from build123d import *

# Parameters (mm, degrees)
EXTRUDE_1_DEPTH          = 3
SKETCH_2_R               = 7.1
SKETCH_2_R_2             = 5.05
CUT_EXTRUDE_1_DEPTH      = 10
SKETCH_3_R               = 2.55
CUT_EXTRUDE_2_DEPTH      = 10
PATTERN_CIRCULAR_1_COUNT = 3
CHAMFER_1_SIZE           = 0.5
SKETCH_4_R               = 8.1
CUT_EXTRUDE_3_DEPTH      = 1


with BuildPart() as part:
    # 草图1 → 凸台-拉伸1 (new body)
    with BuildSketch(Plane(origin=(0, 0, 0), x_dir=(0, 0, -1), z_dir=(1, 0, 0))):
        with BuildLine():
            ThreePointArc((6.766526321, -35.674580026), (11.667792815, -16.687604516), (9.596471541, 2.812069339))
            ThreePointArc((9.596471541, 2.812069339), (0.889352151, 9.960374127), (-8.946463525, 4.467750037))
            Line((-8.946463525, 4.467750037), (-22.078912993, -21.829374729))
            ThreePointArc((-22.078912993, -21.829374729), (-14.688022315, -43.402261843), (6.766526321, -35.674580026))
        make_face()
    extrude(amount=EXTRUDE_1_DEPTH)

    # 草图2 → 切除-拉伸1 (cut)
    with BuildSketch(Plane.ZY):
        Circle(SKETCH_2_R)
        with Locations((7.764571353, -28.977774789)):
            Circle(SKETCH_2_R_2)
    extrude(amount=-CUT_EXTRUDE_1_DEPTH, mode=Mode.SUBTRACT)

    # 草图3 → 切除-拉伸2 (cut)
    with BuildSketch(Plane.ZY):
        with Locations((5.176380902, -19.318516526)):
            Circle(SKETCH_3_R)
    cut_extrude_2 = extrude(amount=-CUT_EXTRUDE_2_DEPTH, mode=Mode.SUBTRACT)

    # 阵列(圆周)1: 切除-拉伸2 ×3 about axis
    pattern_circular_1_axis = Axis((0, -28.977774789, 7.764571353), (1, 0, 0))
    for i in range(1, PATTERN_CIRCULAR_1_COUNT):
        add(cut_extrude_2.rotate(pattern_circular_1_axis, i * 360 / PATTERN_CIRCULAR_1_COUNT), mode=Mode.SUBTRACT)

    # 倒角1
    chamfer_1_edges = [part.edges().sort_by_distance(p)[0] for p in [
        (3, -28.977774789, 2.714571353),
    ]]
    chamfer(chamfer_1_edges, length=CHAMFER_1_SIZE)

    # 草图4 → 切除-拉伸3 (cut)
    with BuildSketch(Plane.ZY.offset(-3)):
        Circle(SKETCH_4_R)
    extrude(amount=CUT_EXTRUDE_3_DEPTH, mode=Mode.SUBTRACT)


solid = part.part
Read the model definition and answer for the solid it produces. Units are mm, in the model's axes. A direction names the side the tool comes from. Give positions to 0.01 mm unless a question says otherwise; leave off trailing zeros. Write each loop counter-clockwise with the first axis right and the second up, starting at its lowest first coordinate (ties: lowest second). Pieces come first, ordered by that corner, then holes. Notation, with made-up numbers: (-8, 29.25) - (34, 29.25) arc R10 cw to (34, 35.25) - close; hole circle Ø10 at (72, 26). An arc over 180 degrees is marked (long way). Use CSV: the item, a comma, the result in double quotes. Start each with the question number.
(1) Given P1, Ø4, axis at y = -21, z = 14, coming from the -X side; P2, Ø1.5, axis at x = 2, z = -5.5, coming from the +Y side; P3, Ø1, axis at x = 1.5, z = -4, coming from the -Y side, each flat-ended and moving along its own axis, determine where each tip first touches the part or whether it passes through.
(2) Find section D-D (z = -6). Give the vertices of the cut face in (x, y), plus the area to 3 significant figures.
(3) Determine the mould class of faces 3 (the cylindrical face through (1.479, 9.944, -1.056)), 4 (the flat face through (1.479, -8.497, 15.421)), 5 (the cylindrical face through (1.479, -16.963, -11.647)), 6 (the cylindrical face through (1.479, -29.416, 18.795)) for opening direction Z: +Z half, -Z half, draft (parallel to the pull), parting line (faces both ways), or undercut.
(4) Find section C-C (x = 0.55). Give the vertices of the cut face in (y, z).
(5) Consider line 1 along Y through (x, z) = (2.15, 3.5); line 2 along Y through (x, z) = (1.05, 4.5); line 3 along Y through (x, z) = (1.95, -1). Determine where each line is inside the solid, lowest interval first.
(6) Find section A-A (y = 0). Give the vertices of the cut face in (x, z).
(7) Find section B-B (z = 0). Give the vertices of the cut face in (x, y), plus the area to 3 significant figures.
(8) For faces 1 (the cylindrical face through (0.99, 7.04, -0.92)), 2 (the cylindrical face through (2.507, -7.907, -1.756)), determine the directions among +Z, -Z, +X, -X, +Y, -Y from which every point of the face is accessible in a straight line to the end or side of a thin tool.
Findings below:
1,P1,"x = 0"
1,P2,"y = 8.8"
1,P3,"y = -40.34"
2,outline,"(0, -37.13) - (3, -37.13) - (3, -5.44) - (2, -5.44) - (2, -3.8) - (0, -3.8) - close; (0, 3.8) - (2, 3.8) - (2, 5.44) - (3, 5.44) - (3, 8) - (0, 8) - close"
2,area,"109 mm2"
3,face 3,"parting line"
3,face 4,"+Z half"
3,face 5,"-Z half"
3,face 6,"undercut"
4,outline,"(-35.67, -6.77) arc R55 ccw to (2.81, -9.6) arc R10 ccw to (4.47, 8.95) - (-21.83, 22.08) arc R16 ccw (long way) to start; hole circle Ø5.1 at (-36.05, 0.69); hole circle Ø5.1 at (-31.57, 17.42); hole circle Ø10.1 at (-28.98, 7.76); hole circle Ø5.1 at (-19.32, 5.18); hole circle Ø14.2 at (0, 0)"
5,line 1,"-44.4 to -31.68, -26.27 to -21.24, -17.4 to -7.3, 7.3 to 9.37"
5,line 2,"-44.64 to -32.83, -25.12 to -21.78, -16.86 to -5.49, 5.49 to 8.93"
5,line 3,"-42.36 to -37.96, -34.14 to -7.03, 7.03 to 9.95"
6,outline,"(0, -10.34) - (3, -10.34) - (3, -8.1) - (2, -8.1) - (2, -7.1) - (0, -7.1) - close; (0, 7.1) - (2, 7.1) - (2, 8.1) - (3, 8.1) - (3, 11.18) - (0, 11.18) - close"
7,outline,"(0, -42.97) - (3, -42.97) - (3, -38.5) - (0, -38.5) - close; (0, -33.59) - (3, -33.59) - (3, -8.1) - (2, -8.1) - (2, -7.1) - (0, -7.1) - close; (0, 7.1) - (2, 7.1) - (2, 8.1) - (3, 8.1) - (3, 10) - (0, 10) - close"
7,area,"99.6 mm2"
8,face 1,"+X, -X"
8,face 2,"+X"
